from build123d import *

# Parameters (mm, degrees)
F0_R     = 38.1
F1_DEPTH = 19.05
F2_R     = 19.336038
F3_DEPTH = 19.05
F4_R     = 9.523462
F5_DEPTH = 38.101


with BuildPart() as f1:
    # F0 (on Front) → F1 (new body)
    with BuildSketch(Plane.XZ):
        Circle(F0_R)
    extrude(amount=F1_DEPTH)

    # F2 (on face) → F3 (join)
    with BuildSketch(Plane(origin=(0, 0, 0), x_dir=(-1, 0, 0), z_dir=(0, 1, 0))):
        Circle(F2_R)
    extrude(amount=F3_DEPTH)

    # F4 (on face) → F5 (cut, through all)
    with BuildSketch(Plane(origin=(0, 19.05, 0), x_dir=(-1, 0, 0), z_dir=(0, 1, 0))):
        Circle(F4_R)
    extrude(amount=-F5_DEPTH, mode=Mode.SUBTRACT)


solid = f1.part
CAD build for the part. Positions are in the model's coordinates, mm. A direction names the side the tool comes from. Coordinates: 2 decimals unless noted, no trailing zeros. Write each loop counter-clockwise with the first axis right and the second up, starting at its lowest first coordinate (ties: lowest second). Pieces come first, ordered by that corner, then holes. Notation, with made-up numbers: (33.25, -33.5) - (89.25, -33.5) arc R34 cw to (89.25, 1.5) - close; hole circle Ø10 at (-17.5, -30.75). An arc over 180 degrees is marked (long way). Use a Markdown table: item, result. Add a question column.
Item 1: Band-saw the part on B-B, the plane z = 0. Give the cut face in (x, y), and give its area (3 significant figures).
Item 2: Band-saw the part on A-A, the plane x = 0. Give the cut face in (y, z), and give its area (3 significant figures).
Item 3: Band-saw the part on D-D, the plane x = -10.5. Give the cut face in (y, z).
Item 4: Flat gauge pins, fed straight in: pin 1 (4 mm diameter, centred on x = 10, y = 13, fed in from -Z); pin 2 (3 mm diameter, centred on y = -10, z = -19.5, fed in from +X); pin 3 (8 mm diameter, centred on y = 13.5, z = 19, fed in from +X). Where does each tip first touch, or does it go through?
Item 5: Drill centre lines: L1, parallel to Z at x = 0, y = -7; L2, parallel to Z at x = 0, y = 7; L3, parallel to Y at x = -35, z = 2.5. Where is each one in solid material? Low to high. Write a range as from..to.
Item 6: Band-saw the part on C-C, the plane y = -15.5. Give the cut face in (x, z), and give its area (3 significant figures).
Item 7: Mould opens along X. For faces 1 (the face through (-30.235, -9.392, -23.183)), 2 (the face through (2.06, 0.27, -9.3)), 3 (the face through (8, -19.05, -8)) say: pulls with the +X half, pulls with the -X half, needs draft (parallel to the pull), parting line crosses it, or undercut.
Item 8: 3-axis set-ups, long thin cutter, end or side, ignore diameter. For faces 4 (the face through (-4, 19.05, 9)), 5 (the face through (-17.5, 0, 9)): which of +Z, -Z, +X, -X, +Y, -Y reach the whole face in a straight line?
Numbers:
| question | item | result |
|---|---|---|
| 1 | outline | (-38.1, -19.05) - (-9.52, -19.05) - (-9.52, 19.05) - (-19.34, 19.05) - (-19.34, 0) - (-38.1, 0) - close; (9.52, -19.05) - (38.1, -19.05) - (38.1, 0) - (19.34, 0) - (19.34, 19.05) - (9.52, 19.05) - close |
| 1 | area | 1,460 mm2 |
| 2 | outline | (-19.05, -38.1) - (0, -38.1) - (0, -19.34) - (19.05, -19.34) - (19.05, -9.52) - (-19.05, -9.52) - close; (-19.05, 9.52) - (19.05, 9.52) - (19.05, 19.34) - (0, 19.34) - (0, 38.1) - (-19.05, 38.1) - close |
| 2 | area | 1,460 mm2 |
| 3 | outline | (-19.05, -36.62) - (0, -36.62) - (0, -16.24) - (19.05, -16.24) - (19.05, 16.24) - (0, 16.24) - (0, 36.62) - (-19.05, 36.62) - close |
| 4 | pin 1 | z = -17.6 |
| 4 | pin 2 | x = 33.58 |
| 4 | pin 3 | x = 12.2 |
| 5 | L1 | -38.1..-9.52, 9.52..38.1 |
| 5 | L2 | -19.34..-9.52, 9.52..19.34 |
| 5 | L3 | -19.05..0 |
| 6 | outline | circle Ø76.2 at (0, 0); hole circle Ø19.05 at (0, 0) |
| 6 | area | 4,280 mm2 |
| 7 | face 1 | parting line crosses it |
| 7 | face 2 | undercut |
| 7 | face 3 | needs draft |
| 8 | face 4 | +Z, -Z, +X, -X, +Y |
| 8 | face 5 | +Y |
